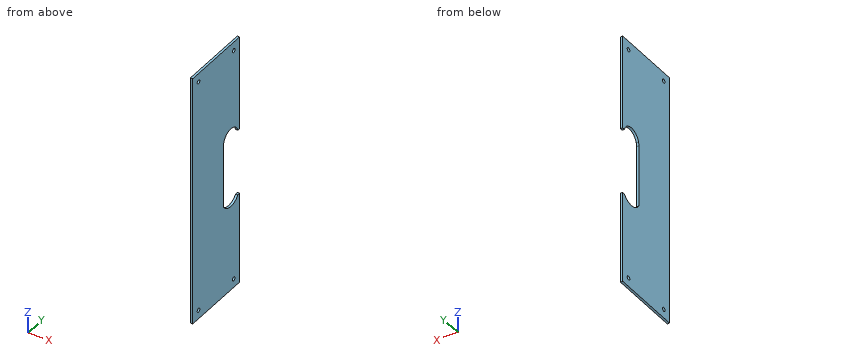
Autodesk Inventor part; units mm, degrees
ref_plane "YZ Plane" through (0, 0, 0) normal (1, 0, 0) x (0, 1, 0)
ref_plane "XZ Plane" through (0, 0, 0) normal (0, 1, 0) x (-1, 0, 0)
ref_plane "XY Plane" through (0, 0, 0) normal (0, 0, 1) x (1, 0, 0)
sketch "スケッチ1" plane through (0, 0, 0) normal (1, 0, 0) x (0, 1, 0)
  line L0 (125.6523, 179.1954) -> (45.6523, 179.1954)
  line L1 (45.6523, 179.1954) -> (45.6523, -110.8046)
  line L2 (45.6523, -110.8046) -> (125.6523, -110.8046)
  line L3 (125.6523, -110.8046) -> (125.6523, 179.1954)
  point P0 (0, 0)
  dimension "d0" = 80
  dimension "d1" = 290
extrude "押し出し1" add sketch "スケッチ1" along normal blind 2.6
sketch "スケッチ2" plane through (2.6, 0, 0) normal (1, 0, 0) x (0, 0, -1)
  line L0 (-179.1954, 125.6523) -> (-179.1954, 45.6523)
  line L1 (-179.1954, 45.6523) -> (110.8046, 45.6523)
  line L2 (110.8046, 45.6523) -> (110.8046, 125.6523)
  line L3 (110.8046, 125.6523) -> (-179.1954, 125.6523)
  line L4 (-34.1954, 85.6523) -> (-34.1954, 125.6523)
  line L5 (110.8046, 125.6523) -> (-179.1954, 125.6523)
  line L6 (-34.1954, 85.6523) -> (110.8046, 85.6523)
  point P0 (0, 0)
  point P1 (-169.1954, 115.6523)
  point P2 (100.8046, 115.6523)
  point P3 (-169.1954, 55.6523)
  point P4 (100.8046, 55.6523)
  dimension "d4" = 10
  dimension "d5" = 10
hole "穴1" at (2.6, 115.6523, 169.1954) at (2.6, 115.6523, -100.8046) at (2.6, 55.6523, 169.1954) at (2.6, 55.6523, -100.8046) direction (-1, 0, 0) diameter 4.5 depth 10 tip angle 118
sketch "スケッチ4" plane through (0, 0, 0) normal (-1, 0, 0) x (0, 0, 1)
  ellipse E0 centre (2.4593, 110.6523) end of major axis (2.4593, 125.1521) minor radius 14.4996 (-5.7266, 122.6204) -> (-6.1243, 98.9661) ccw
  line L0 (-5.7266, 125.6523) -> (-5.7266, 122.6204)
  line L1 (-4.4935, 97.7683) -> (66.6998, 97.7683)
  line L2 (66.6998, 97.7683) -> (70.683, 98.6842)
  ellipse E1 centre (67.383, 110.6523) end of major axis (67.383, 123.067) minor radius 12.4145 (70.683, 98.6842) -> (70.683, 122.6204) ccw
  line L3 (70.683, 122.6204) -> (70.683, 125.6523)
  ellipse E2 centre (67.383, 110.6523) end of major axis (67.383, 123.067) minor radius 12.4145 (70.683, 98.6842) -> (70.683, 122.6204) ccw
  line L4 (-6.1243, 98.9661) -> (-4.4935, 97.7683)
  line L5 (-110.8046, 125.6523) -> (179.1954, 125.6523)
  arc A0 (66.6955, 101.0165) -> (66.6955, 120.2881) centre (66.6954, 110.6523) ccw
  arc A1 (1.6954, 120.1437) -> (1.6954, 101.1609) centre (1.6954, 110.6523) ccw
  line L6 (1.6954, 120.1437) -> (66.6955, 120.2881)
  line L7 (66.6955, 101.0165) -> (1.6954, 101.1609)
  line L8 (1.6954, 120.1437) -> (1.6954, 125.6523)
  line L9 (-110.8046, 125.6523) -> (179.1954, 125.6523)
  line L10 (66.6955, 120.2881) -> (66.6955, 125.6523)
  point P0 (0, 0)
extrude "押し出し3" cut sketch "スケッチ4" against normal through all
properties part number "lc_box_side" material "ポリカーボネート、クリア"
Geometry: final body of the model. Coordinates: model frame, mm. Round coordinates to 2 decimals unless told otherwise and drop trailing zeros. Loops run counter-clockwise (first coordinate to the right, second up) from the corner with the lowest first, then second, coordinate; pieces in that order, holes last.
Q1. Section A-A on x = 2.15. State how many separate pieces and enclosed holes the cut face has, plus the area to 3 significant figures.
Q2. Material intervals for L1, parallel to Y at x = 2.2, z = 22.5, sorted ascending.
Q3. Section B-B on z = -2. Return loops of the section in (x, y), plus the area to 3 significant figures.
Evaluation:
1. separate pieces: 1
1. enclosed holes: 4
1. area: 20,700 mm2
2. L1: y = 45.65 to 97.77
3. outline: (0, 45.65) - (2.6, 45.65) - (2.6, 97.77) - (0, 97.77) - close
3. area: 136 mm2
